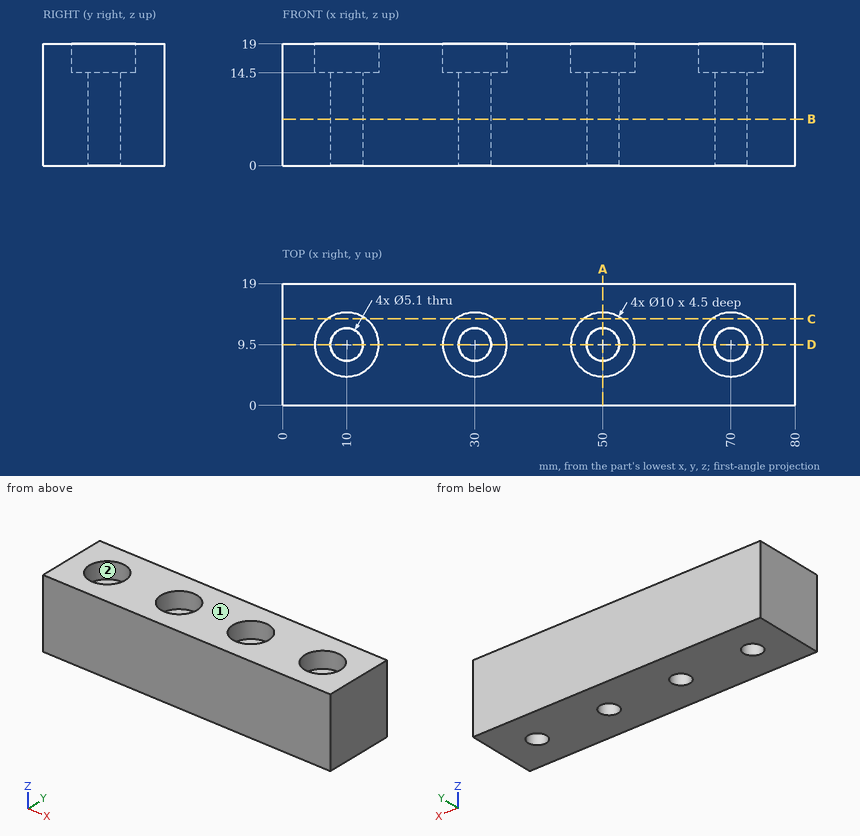
The drawing under review shows one solid part. Ordinate dimensions are in mm from its lowest x, y, z. A direction names the side the tool comes from. Give positions to 0.01 mm unless a question says otherwise; leave off trailing zeros. Order: outer loops, then holes, each group sorted by start corner. A loop starts at its lowest first (then second) coordinate and runs counter-clockwise, first axis right, second up. Notation, with made-up numbers: (66, 39) -> (107, 39) arc R13 ccw to (107, 47) -> close; hole circle Ø8 at (3, -24). An arc over 180 degrees is marked (long way). Write item = value, one per line. Start each with the question number.
(1) For the marked faces 1 and 2, list the 3-axis set-ups (+Z, -Z, +X, -X, +Y, -Y) from which the entire face can be reached by the end or side of a thin tool; tool diameter is ignored.
(2) We need section A-A on x = 50. Write out the cut boundary in (y, z).
(3) To check wall thickness, follow line 1 along X through (y, z) = (9.5, 6.75); line 2 along Y through (x, z) = (10, 15.75); line 3 along Y through (x, z) = (70, 5). State the ranges of each line that lie inside material, in increasing order.
(4) We need section D-D on y = 9.5. State how many separate pieces and enclosed holes the cut face has, plus the area to 3 significant figures.
(5) For pin 1 (4 mm diameter, centred on x = 50, y = 9.5, fed in from +Z); pin 2 (9 mm diameter, centred on x = 30, y = 9.5, fed in from +Z), all flat-tipped, find the tip position at first contact; note any pin that passes through.
(6) We need section C-C on y = 13.5. Write out the cut boundary in (x, z), plus the area to 3 significant figures.
(7) We need section B-B on z = 7.25. Write out the cut boundary in (x, y), plus the area to 3 significant figures.
Numbers:
q1.face_1 = +Z, +X, -X, +Y, -Y
q1.face_2 = +Z
q2.outline = (0, 0) -> (6.95, 0) -> (6.95, 14.5) -> (4.5, 14.5) -> (4.5, 19) -> (0, 19) -> close; (12.05, 0) -> (19, 0) -> (19, 19) -> (14.5, 19) -> (14.5, 14.5) -> (12.05, 14.5) -> close
q3.line_1 = 0 to 7.45, 12.55 to 27.45, 32.55 to 47.45, 52.55 to 67.45, 72.55 to 80
q3.line_2 = 0 to 4.5, 14.5 to 19
q3.line_3 = 0 to 6.95, 12.05 to 19
q4.separate_pieces = 5
q4.enclosed_holes = 0
q4.area = 1,040 mm^2
q5.pin_1 = through
q5.pin_2 = 14.5
q6.outline = (0, 0) -> (80, 0) -> (80, 19) -> (73, 19) -> (73, 14.5) -> (67, 14.5) -> (67, 19) -> (53, 19) -> (53, 14.5) -> (47, 14.5) -> (47, 19) -> (33, 19) -> (33, 14.5) -> (27, 14.5) -> (27, 19) -> (13, 19) -> (13, 14.5) -> (7, 14.5) -> (7, 19) -> (0, 19) -> close
q6.area = 1,410 mm^2
q7.outline = (0, 0) -> (80, 0) -> (80, 19) -> (0, 19) -> close; hole circle Ø5.1 at (10, 9.5); hole circle Ø5.1 at (30, 9.5); hole circle Ø5.1 at (50, 9.5); hole circle Ø5.1 at (70, 9.5)
q7.area = 1,440 mm^2
